```python
from build123d import *

# Parameters (mm, degrees)
BOSS_EXTRUDE1_DEPTH = 15
FILLET1_R           = 2


with BuildPart() as part:
    # Sketch1 → Boss-Extrude1 (new body)
    with BuildSketch(Plane(origin=(0, 0, 0), x_dir=(1, 0, 0), z_dir=(0, 1, 0))):
        with BuildLine():
            Line((0, 0), (0, 7))
            Line((0, 7), (12, 7))
            ThreePointArc((12, 7), (16.949747468, 4.949747468), (19, 0))
            Line((19, 0), (19, -8))
            Line((19, -8), (15, -8))
            Line((15, -8), (15, -6))
            Line((15, -6), (11, -6))
            Line((11, -6), (11, -12))
            Line((11, -12), (23, -12))
            Line((23, -12), (23, 0))
            ThreePointArc((23, 0), (19.778174593, 7.778174593), (12, 11))
            Line((12, 11), (-4, 11))
            Line((-4, 11), (-4, 0))
            Line((-4, 0), (0, 0))
        make_face()
    extrude(amount=BOSS_EXTRUDE1_DEPTH)

    # Fillet1
    fillet1_edges = [part.edges().sort_by_distance(p)[0] for p in [
        (15, 7.5, 6),
        (0, 7.5, 0),
        (-4, 7.5, -11),
    ]]
    fillet(fillet1_edges, radius=FILLET1_R - 0.0001)  # a hair under: the kernel refuses the full size


solid = part.part
```
Source: CAD feature listing. Evaluate the final solid. Frame: model axes, mm. A direction names the side the tool comes from. Round coordinates to 2 decimals unless told otherwise and drop trailing zeros. Loops run counter-clockwise (first coordinate to the right, second up) from the corner with the lowest first, then second, coordinate; pieces in that order, holes last. Notation, with made-up numbers: M 10,55 L 43,55 A20 cw 43,78 Z; hole C -16.5,-7 d3. An arc over 180 degrees is marked long. Use a Markdown table: item, result. Add a question column.
1. Pull-direction query (Z, two-part tool) for faces 4 (the cylindrical face through (-0.57, 7.6, -0.6)), 5 (the cylindrical face through (-3.4, 7.6, -10.43)), 6 (the flat face through (19, 7, 4)); classes: +Z half, -Z half, draft (parallel to the pull), parting line (faces both ways), or undercut.
2. Cut plane A-A, the plane x = 16.25. Output: boundary loops of the cut face in (y, z).
3. Set-up query: faces 1 (the cylindrical face through (16.9, 7.4, -5)), 2 (the flat face through (12, 7, 6)), 3 (the flat face through (11, 7, 9)). Return all of +Z, -Z, +X, -X, +Y, -Y with unobstructed straight access to the full face (end or side cutting, diameter ignored); none if empty.
4. Contact query for flat-ended pins moving along their axis: pin 1 (0.6 mm diameter, centred on x = -3, y = 5.5, fed in from +Z); pin 2 (4 mm diameter, centred on y = 7, z = -5, fed in from +X); pin 3 (3 mm diameter, centred on x = 17.5, y = 6, fed in from -Z). Output: stop coordinate, or through.
5. Ray query, line 1 along Z through (x, y) = (12.25, 1.5); line 2 along X through (y, z) = (2.25, 10.5); line 3 along X through (y, z) = (5.5, -4.5). Return the intervals inside material, ascending. Write a range as [from, to].
6. Cut plane D-D, the plane z = 0.75. Output: boundary loops of the cut face in (x, y).
7. Cut plane B-B, the plane z = -5.25. Output: boundary loops of the cut face in (x, y), and give its area (3 significant figures).
Solution:
| question | item | result |
|---|---|---|
| 1 | face 4 | +Z half |
| 1 | face 5 | -Z half |
| 1 | face 6 | undercut |
| 2 | outline | M 0,-10.15 L 15,-10.15 L 15,-5.56 L 0,-5.56 Z; M 0,8 L 15,8 L 15,12 L 0,12 Z |
| 3 | face 1 | +Y, -Y |
| 3 | face 2 | -X, +Y, -Y |
| 3 | face 3 | +Z, -X, +Y, -Y |
| 4 | pin 1 | stops at z = 0 |
| 4 | pin 2 | stops at x = 22.58 |
| 4 | pin 3 | stops at z = -10.25 |
| 5 | line 1 | z = [-11, -7], [6, 12] |
| 5 | line 2 | x = [11, 23] |
| 5 | line 3 | x = [-4, 0], [17.36, 22.04] |
| 6 | outline | M 19,0 L 23,0 L 23,15 L 19,15 Z |
| 7 | outline | M -4,0 L 0,0 L 0,15 L -4,15 Z; M 16.63,0 L 21.67,0 L 21.67,15 L 16.63,15 Z |
| 7 | area | 136 mm2 |
